```python
from build123d import *

# Parameters (mm, degrees)
SKETCH2_R           = 5
BOSS_EXTRUDE1_DEPTH = 15


with BuildPart() as part:
    # Sketch2 → Boss-Extrude1 (new body)
    with BuildSketch(Plane(origin=(0, 340, 0), x_dir=(1, 0, 0), z_dir=(0, 1, 0))):
        Polygon((-420.637885724, -681.858342538), (-30.637885724, -681.858342538), (-30.637885724, -455.858342538), (-30.637885724, -433.881423439), (-420.637885724, -433.881423439), (-420.637885724, -455.858342538), align=None)
        with Locations(Location((-53.137885724, -493.881423439, 0), (0, 0, 180))):
            Circle(SKETCH2_R, mode=Mode.SUBTRACT)
        with Locations((-53.137885724, -622.094154379)):
            Circle(SKETCH2_R, mode=Mode.SUBTRACT)
        with Locations((-398.137885724, -493.881423439)):
            Circle(SKETCH2_R, mode=Mode.SUBTRACT)
        with Locations(Location((-398.137885724, -622.094154379, 0), (0, 0, 180))):
            Circle(SKETCH2_R, mode=Mode.SUBTRACT)
        with Locations(Location((-197.384432093, -549.451182731, 0), (0, 0, 180))):
            Circle(SKETCH2_R, mode=Mode.SUBTRACT)
        with Locations(Location((-197.384432093, -606.081360459, 0), (0, 0, 180))):
            Circle(SKETCH2_R, mode=Mode.SUBTRACT)
        with Locations(Location((-253.891339355, -606.081360459, 0), (0, 0, 180))):
            Circle(SKETCH2_R, mode=Mode.SUBTRACT)
        with Locations(Location((-253.891339355, -549.451182731, 0), (0, 0, 180))):
            Circle(SKETCH2_R, mode=Mode.SUBTRACT)
    extrude(amount=BOSS_EXTRUDE1_DEPTH)


solid = part.part
```
The listing builds one solid part. Answer for the finished solid, in the listing's coordinates (mm). Coordinates: 2 decimals unless noted, no trailing zeros. Use a Markdown table: item, result. Add a question column.
1) The mould has two halves that part along X. Classify faces 1 (the flat face through (-420.638, 347, 556)), 2 (the cylindrical face through (-400.826, 347.395, 626.31)), 3 (the flat face through (-228, 340, 556)): released by +X, released by -X, zero draft, split by the parting line, or undercut.
2) Given pin 1 (9 mm diameter, centred on x = -53.14, z = 622.09, fed in from -Y), flat-ended and moving along its own axis, determine where the tip first touches the part or whether it passes through.
3) Find the intervals of material crossed by line 1 (X direction, y = 348, z = 603), in increasing order.
Here are the results:
| question | item | result |
|---|---|---|
| 1 | face 1 | released by -X |
| 1 | face 2 | undercut |
| 1 | face 3 | zero draft |
| 2 | pin 1 | passes through |
| 3 | line 1 | x = -420.64 to -257.83, -249.95 to -201.32, -193.45 to -30.64 |
